Verification items for the finished model (mm, model axes). Face numbers are marked on the shaded views. A direction names the side the tool comes from. Round coordinates to 2 decimals unless told otherwise and drop trailing zeros. Loops run counter-clockwise (first coordinate to the right, second up) from the corner with the lowest first, then second, coordinate; pieces in that order, holes last. Notation, with made-up numbers: M 33,-28.75 L 81,-28.75 A24 cw 81,9.25 Z; hole C 61,88.25 d9. An arc over 180 degrees is marked long. Answer as CSV lines item,"result".
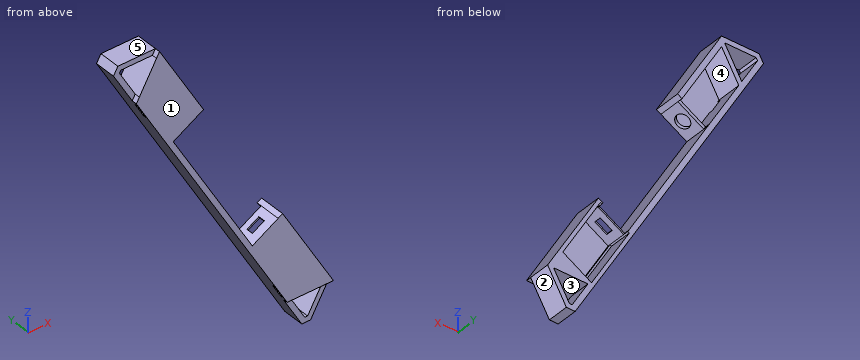
```python
from build123d import *

# Parameters (mm, degrees)
BOSS_EXTRUDE2_DEPTH = 15.38
BOSS_EXTRUDE3_DEPTH = 1
BOSS_EXTRUDE4_DEPTH = 12.38
CUT_EXTRUDE1_DEPTH  = 8.26
SKETCH12_R          = 4
CUT_EXTRUDE2_DEPTH  = 8.26
CUT_EXTRUDE3_DEPTH  = 3
SKETCH16_W          = 10
SKETCH16_H          = 2
CUT_EXTRUDE4_DEPTH  = 3
CUT_EXTRUDE5_DEPTH  = 13


with BuildPart() as part:
    # Sketch1 → Boss-Extrude2 (new body)
    with BuildSketch(Plane(origin=(0, 0, 0), x_dir=(1, 0, 0), z_dir=(0, 1, 0))):
        Polygon((-33.232050802, 130.626242439), (-11.732050802, 167.865334802), (3.267949197, 159.205080764), (-18.232050803, 121.965988402), (-18.732050803, 121.099962998), (-16.133974592, 119.599962998), (13.464101619, 170.865334801), (2.556624332, 189.757639644), (-2.556624322, 189.757639644), (-112.11324865, 2e-09), (-109.556624323, -4.428203228), (-87.74166975, -4.428203228), (-62.14359354, 39.908965344), (-64.74166975, 41.408965344), (-65.74166975, 39.676914536), (-82.74166975, 10.232050807), (-87.74166975, 1.57179677), (-97.741669749, 18.892304845), (-80.741669749, 48.337168573), (-79.741669749, 50.069219381), (-33.732050802, 129.760217035), align=None)
        Polygon((-89.473720558, -1.42820323), (-107.824573519, -1.42820323), (-108.649147039, 0), (-99.473720558, 15.892304845), align=None, mode=Mode.SUBTRACT)
        Polygon((-9.999999996, 170.865334801), (-0.824573515, 186.757639646), (0.824573508, 186.757639646), (10.000000004, 170.865334801), align=None, mode=Mode.SUBTRACT)
    extrude(amount=BOSS_EXTRUDE2_DEPTH)

    # Sketch1_11 → Boss-Extrude3 (add)
    with BuildSketch(Plane(origin=(0, 0, 0), x_dir=(1, 0, 0), z_dir=(0, 1, 0))):
        Polygon((3.267949197, 159.205080764), (-11.732050802, 167.865334802), (-33.232050802, 130.626242439), (-18.232050803, 121.965988402), align=None)
        Polygon((-65.74166975, 39.676914536), (-80.741669749, 48.337168573), (-97.741669749, 18.892304845), (-87.74166975, 1.57179677), align=None)
    extrude(amount=BOSS_EXTRUDE3_DEPTH)

    # Sketch1_12 → Boss-Extrude4 (add)
    with BuildSketch(Plane(origin=(0, 0, 0), x_dir=(1, 0, 0), z_dir=(0, 1, 0))):
        Polygon((-33.732050802, 129.760217035), (-33.232050802, 130.626242439), (-18.232050803, 121.965988402), (-18.732050803, 121.099962998), align=None)
        Polygon((-64.74166975, 41.408965344), (-79.741669749, 50.069219381), (-80.741669749, 48.337168573), (-65.74166975, 39.676914536), align=None)
    extrude(amount=BOSS_EXTRUDE4_DEPTH)

    # Sketch10 → Cut-Extrude1 (cut)
    with BuildSketch(Plane(origin=(47.754809476, 0, -82.713756318), x_dir=(0.8660254037844418, 0, 0.49999999999999456), z_dir=(-0.4999999999999946, 0, 0.8660254037844419))):
        Polygon((-85.432921433, 5), (-81.432921433, 5), (-81.432921433, 9), (-89.432921433, 9), (-89.432921433, 5), align=None)
    extrude(amount=-CUT_EXTRUDE1_DEPTH, mode=Mode.SUBTRACT)

    # Sketch12 → Cut-Extrude2 (cut)
    with BuildSketch(Plane(origin=(1.745190528, 0, -3.022758664), x_dir=(-0.866025403784436, 0, -0.5000000000000047), z_dir=(0.5000000000000047, 0, -0.866025403784436))):
        with Locations((85.432921433, 6.5)):
            Circle(SKETCH12_R)
    extrude(amount=-CUT_EXTRUDE2_DEPTH, mode=Mode.SUBTRACT)

    # Sketch15 → Cut-Extrude3 (cut)
    with BuildSketch(Plane.XZ):
        Polygon((-87.74166975, 4.428203228), (-109.556624323, 4.428203228), (-112.11324865, -2e-09), (-101.205771363, -18.892304845), align=None)
        Polygon((13.464101619, -170.865334801), (2.556624332, -189.757639644), (-2.556624322, -189.757639644), (-13.464101609, -170.865334801), align=None)
    extrude(amount=-CUT_EXTRUDE3_DEPTH, mode=Mode.SUBTRACT)

    # Sketch16 → Cut-Extrude4 (cut)
    with BuildSketch(Plane(origin=(-84.084936489, 0, -48.546460716), x_dir=(-0.4999999999999999, 0, 0.8660254037844386), z_dir=(-0.8660254037844387, 0, -0.49999999999999994))):
        with Locations((-133.242624333, 2)):
            Rectangle(SKETCH16_W, SKETCH16_H)
        with Locations((26.242624323, 2)):
            Rectangle(SKETCH16_W, SKETCH16_H)
    extrude(amount=-CUT_EXTRUDE4_DEPTH, mode=Mode.SUBTRACT)

    # Sketch17 → Cut-Extrude5 (cut)
    with BuildSketch(Plane(origin=(0, 15.38, 0), x_dir=(1, 0, 0), z_dir=(0, 1, 0))):
        Polygon((-18.232050803, 121.965988402), (-17.366025399, 121.465988402), (4.633974601, 159.571106168), (-12.098076205, 169.231360205), (-34.098076205, 131.126242439), (-33.232050802, 130.626242439), align=None)
    extrude(amount=-CUT_EXTRUDE5_DEPTH, mode=Mode.SUBTRACT)


solid = part.part
```
1) Section check D-D (z = -113.5). Record the cut outline in (x, y).
Here are the results:
outline,"M -46.58,0 L -43.12,0 L -43.12,15.38 L -46.58,15.38 Z"
2) Section check C-C (x = -46). Record the cut outline in (y, z).
Here are the results:
outline,"M 0,-114.51 L 15.38,-114.51 L 15.38,-108.51 L 0,-108.51 Z"
3) Draft check along X on the marked faces 1, 2 and 3. Enter one of: +X half, -X half, draft (parallel to the pull), parting line (faces both ways), or undercut.
Here are the results:
face 1,"draft"
face 2,"+X half"
face 3,"undercut"
4) Go/stop test with flat-tipped pins: pin 1 (1.8 mm diameter, centred on x = 0, y = 11.5, fed in from +Z); pin 2 (8 mm diameter, centred on x = -59.5, z = -34.5, fed in from -Y); pin 3 (25 mm diameter, centred on x = -5.5, z = -142.5, fed in from +Y); pin 4 (5.5 mm diameter, centred on x = -25, z = -125, fed in from +Y). Record where each tip stops, or that it passes through.
Here are the results:
pin 1,"stops at z = -145.99"
pin 2,"passes through"
pin 3,"stops at y = 15.38"
pin 4,"stops at y = 12.38"
5) Section check A-A (z = -175.5). Record the cut outline in (x, y), plus the area to 3 significant figures.
Here are the results:
outline,"M -10.79,3 L -7.32,3 L -7.32,15.38 L -10.79,15.38 Z; M 7.32,3 L 10.79,3 L 10.79,15.38 L 7.32,15.38 Z"
area,"85.8 mm^2"
6) Section check B-B (z = -138). Record the cut outline in (x, y).
Here are the results:
outline,"M -32.44,0 L -5.51,0 L -5.51,15.38 L -7.82,15.38 L -7.82,2.38 L -8.97,2.38 L -8.97,1 L -28.97,1 L -28.97,2.38 L -30.13,2.38 L -30.13,15.38 L -32.44,15.38 Z"
7) Set-up check for the marked faces 4 and 5: record each of +Z, -Z, +X, -X, +Y, -Y from which the full face is reachable in a straight line by a thin tool's end or side.
Here are the results:
face 4,"+Y"
face 5,"+Z, +X, -X, +Y, -Y"
8) Material ranges on probe 1 along Z at (x, y) = (-5.5, 5.75); probe 2 along Z at (x, y) = (-93, 9); probe 3 along Y at (x, z) = (-88, -32), recorded low to high.
Here are the results:
probe 1,"z = -184.66 to -178.66, -170.87 to -165.42, -142.02 to -138.02"
probe 2,"z = -33.11 to -27.11, -10.68 to -4.68, 1.43 to 4.43"
probe 3,"y = 0 to 1"
